Job drawing, mm, ordinate dimensions from the low corner. One solid piece. Give positions to 0.01 mm unless a question says otherwise; leave off trailing zeros. Loops run counter-clockwise (first coordinate to the right, second up) from the corner with the lowest first, then second, coordinate; pieces in that order, holes last. Notation, with made-up numbers: (-25, 24) -> (-4, 24) arc R12 cw to (-4, 42) -> close; hole circle Ø7 at (57, 69). An arc over 180 degrees is marked (long way). Use one line per item in the form item = value.
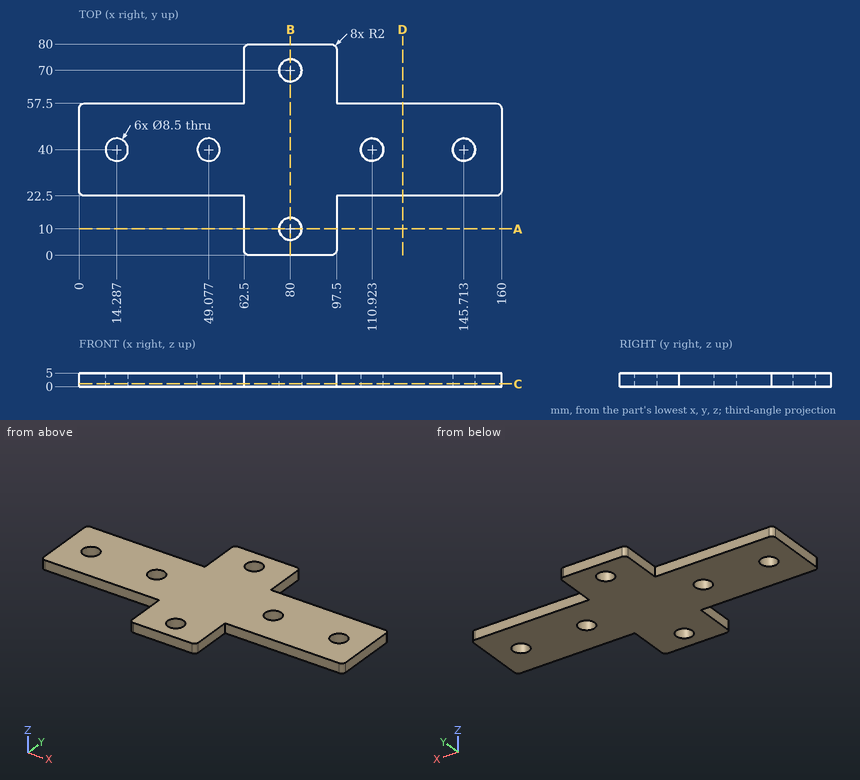
1. Cut at D-D, the plane x = 122.5. Write the cut outline in (y, z).
Result sheet:
outline = (22.5, 0) -> (57.5, 0) -> (57.5, 5) -> (22.5, 5) -> close
2. Cut at C-C, the plane z = 1.05. Write the cut outline in (x, y), then the cut area to 3 significant figures.
Result sheet:
outline = (0, 24.5) arc R2 ccw to (2, 22.5) -> (62.5, 22.5) -> (62.5, 2) arc R2 ccw to (64.5, 0) -> (95.5, 0) arc R2 ccw to (97.5, 2) -> (97.5, 22.5) -> (158, 22.5) arc R2 ccw to (160, 24.5) -> (160, 55.5) arc R2 ccw to (158, 57.5) -> (97.5, 57.5) -> (97.5, 78) arc R2 ccw to (95.5, 80) -> (64.5, 80) arc R2 ccw to (62.5, 78) -> (62.5, 57.5) -> (2, 57.5) arc R2 ccw to (0, 55.5) -> close; hole circle Ø8.5 at (14.29, 40); hole circle Ø8.5 at (49.08, 40); hole circle Ø8.5 at (80, 10); hole circle Ø8.5 at (80, 70); hole circle Ø8.5 at (110.92, 40); hole circle Ø8.5 at (145.71, 40)
area = 6,830 mm^2
3. Cut at B-B, the plane x = 80. Write the cut outline in (y, z), then the cut area to 3 significant figures.
Result sheet:
outline = (0, 0) -> (5.75, 0) -> (5.75, 5) -> (0, 5) -> close; (14.25, 0) -> (65.75, 0) -> (65.75, 5) -> (14.25, 5) -> close; (74.25, 0) -> (80, 0) -> (80, 5) -> (74.25, 5) -> close
area = 315 mm^2
4. Cut at A-A, the plane y = 10. Write the cut outline in (x, z).
Result sheet:
outline = (62.5, 0) -> (75.75, 0) -> (75.75, 5) -> (62.5, 5) -> close; (84.25, 0) -> (97.5, 0) -> (97.5, 5) -> (84.25, 5) -> close
5. Drop flat-ended pins along their axis: P1, Ø2.5, axis at y = 14.5, z = 3.5, coming from the +X side; P2, Ø11, axis at x = 49.08, y = 40, coming from the +Z side; P3, Ø1.5, axis at y = 56.5, z = 1, coming from the -X side; P4, Ø2.5, axis at x = 117, z = 2, coming from the +Y side. Give the stop position or say it passes through.
Result sheet:
P1 = 97.5
P2 = 5
P3 = 0.02
P4 = 57.5
6. Drill centre lines: line 1 (X direction, y = 10, z = 3.2); line 2 (Y direction, x = 80, z = 1.8); line 3 (Y direction, x = 25, z = 0.7). Where is each one in solid material? Low to high.
Result sheet:
line_1 = 62.5 to 75.75, 84.25 to 97.5
line_2 = 0 to 5.75, 14.25 to 65.75, 74.25 to 80
line_3 = 22.5 to 57.5
